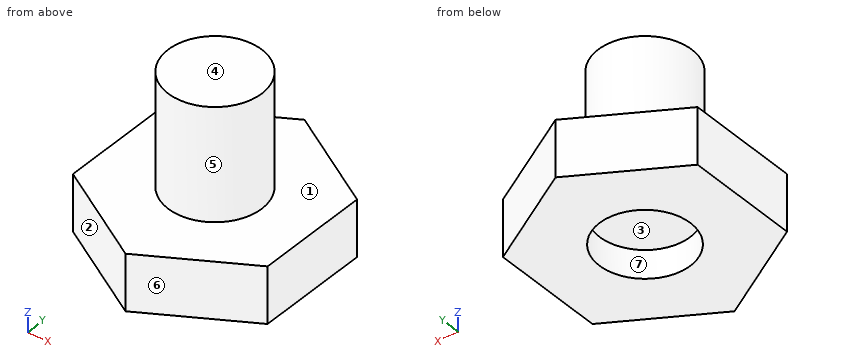
Autodesk Fusion 360 part; units mm, degrees
sketch "Sketch1" plane through (0, 0, 0) normal (0, 0, 1) x (1, 0, 0)
  line L0 (-34.3393, 20.6317) -> (-35.0372, -19.4228)
  line L1 (-35.0372, -19.4228) -> (-0.698, -40.0546)
  line L2 (-0.698, -40.0546) -> (34.3393, -20.6317)
  line L3 (34.3393, -20.6317) -> (35.0372, 19.4228)
  line L4 (35.0372, 19.4228) -> (0.698, 40.0546)
  line L5 (0.698, 40.0546) -> (-34.3393, 20.6317)
extrude "Extrude1" add sketch "Sketch1" along normal blind 20 makes body 1
sketch "Sketch2" plane through (0, 0, 20) normal (0, 0, 1) x (-1, 0, 0)
  line L0 (-0.698, -40.0546) -> (34.3393, -20.6317)
  line L1 (34.3393, -20.6317) -> (35.0372, 19.4228)
  line L2 (35.0372, 19.4228) -> (0.698, 40.0546)
  line L3 (0.698, 40.0546) -> (-34.3393, 20.6317)
  line L4 (-34.3393, 20.6317) -> (-35.0372, -19.4228)
  line L5 (-35.0372, -19.4228) -> (-0.698, -40.0546)
  circle A0 centre (0, 0) radius 16.161
extrude "Extrude2" cut sketch "Sketch2" against normal blind 60 contours A0 bodies 1
sketch "Sketch3" plane through (0, 0, 0) normal (0, 0, 1) x (1, 0, 0)
  circle A0 centre (-100, 0) radius 16.6427
extrude "Extrude3" add sketch "Sketch3" along normal blind 50 separate body makes body 2
thread "Thread1" thread offset 0 thread length 10
move_body "Move1" bodies 2 to x (1, 0, 0) y (0, 1, 0) z (0, 0, 1) at (100, 0, 10)
combine "Combine1" operation add target body 1 tool bodies 2
thread "Thread2" thread offset 0 thread length 10
Geometry: final body of the model. Coordinates: model frame, mm. Face numbers are marked on the shaded views. A direction names the side the tool comes from. Coordinates: 2 decimals unless noted, no trailing zeros. Order: outer loops, then holes, each group sorted by start corner. A loop starts at its lowest first (then second) coordinate and runs counter-clockwise, first axis right, second up.
(1) Section query A-A (y = 11). Return the cut outline in (x, z), plus the area to 3 significant figures.
(2) Material intervals for probe 1 along Z at (x, y) = (16, 27); probe 2 along Z at (x, y) = (1, 0); probe 3 along Y at (x, z) = (0, 3), sorted ascending.
(3) Access query for the marked faces 1, 2 and 3. Directions: +Z, -Z, +X, -X, +Y, -Y. A direction counts if a zero-diameter tool reaches every point of the face in a straight line with its end or side. Return the directions, or none.
(4) First-contact query: pin 1 (1 mm diameter, centred on x = 7, z = 31, fed in from +Y); pin 2 (2 mm diameter, centred on y = 19.5, z = 17, fed in from -X); pin 3 (10 mm diameter, centred on y = 4, z = 39.5, fed in from +X). Flat tips, straight axial feed; report the tip coordinate or a pass-through.
(5) Section query B-B (x = -15). Return the cut outline in (y, z).
(6) Draft query along X for the marked faces 4, 5, 6 and 7. Return one class per face: pulls with the +X half, pulls with the -X half, needs draft (parallel to the pull), parting line crosses it, or undercut.
(7) Section query D-D (z = 27). Return the cut outline in (x, y).
(8) Section query C-C (z = 11.5). Return the cut outline in (x, y).
Solution:
1. outline: (-34.51, 0) - (-11.84, 0) - (-11.84, 10) - (11.84, 10) - (11.84, 0) - (34.89, 0) - (34.89, 20) - (12.49, 20) - (12.49, 60) - (-12.49, 60) - (-12.49, 20) - (-34.51, 20) - close
1. area: 2,150 mm2
2. probe 1: z = 0 to 20
2. probe 2: z = 10 to 60
2. probe 3: y = -39.67 to -16.16, 16.16 to 39.67
3. face 1: +Z
3. face 2: +Z, -Z, -X, -Y
3. face 3: -Z
4. pin 1: stops at y = 15.32
4. pin 2: stops at x = -34.38
4. pin 3: stops at x = 16.64
5. outline: (-31.46, 0) - (-6.01, 0) - (-6.01, 10) - (6.01, 10) - (6.01, 0) - (31.35, 0) - (31.35, 20) - (7.21, 20) - (7.21, 60) - (-7.21, 60) - (-7.21, 20) - (-31.46, 20) - close
6. face 4: needs draft
6. face 5: parting line crosses it
6. face 6: pulls with the +X half
6. face 7: undercut
7. outline: circle Ø33.29 at (0, 0)
8. outline: (-35.04, -19.42) - (-0.7, -40.05) - (34.34, -20.63) - (35.04, 19.42) - (0.7, 40.05) - (-34.34, 20.63) - close
